Autodesk Inventor part; units mm, degrees
ref_plane "YZ Plane" through (0, 0, 0) normal (1, 0, 0) x (0, 1, 0)
ref_plane "XZ Plane" through (0, 0, 0) normal (0, 1, 0) x (-1, 0, 0)
ref_plane "Arbeitsebene1" through (0, 0, -17.5) normal (0, 0, 1) x (1, 0, 0)
sketch "Skizze1" plane through (0, 0, -17.5) normal (0, 0, 1) x (1, 0, 0)
  arc A0 (5.2, -17) -> (15.2, -17) centre (10.2, -17) ccw
  circle A1 centre (10.2, -17) radius 2.3
  circle A2 centre (10.2, 17) radius 2.3
  arc A3 (15.2, 17) -> (5.2, 17) centre (10.2, 17) ccw
  line L0 (15.2, 17) -> (15.2, -17)
  line L1 (5.2, -17) -> (5.2, 17)
  point P0 (0, 0)
  dimension "d17" = 34
  dimension "d19" = 5
  dimension "d20" = 5
  dimension "d21" = 4.6
  dimension "d22" = 4.6
  dimension "d23" = 5.2
  dimension "d24" = 15.2
  dimension "d25" = 17
extrude "Extrusion1" add sketch "Skizze1" against normal blind 20
sketch "Skizze2" plane through (15.2, -17, -17.5) normal (1, 0, 0) x (0, 0, -1)
  circle A0 centre (-2.1, 17) radius 13.4
  circle A1 centre (-2.1, 17) radius 16.4
  line L0 (0, 39) -> (20, 39)
  line L1 (7, 39) -> (7, 30.6437)
  line L2 (7, 39) -> (-2.3022, 41.2587)
  line L3 (-2.3022, 41.2587) -> (-4.5237, 40.7441)
  line L4 (-4.5237, 40.7441) -> (-5.04, 30.0735)
  line L5 (-5.1067, 3.9417) -> (-12.3463, -18.8233)
  line L6 (-12.3463, -18.8233) -> (7.5061, -24.3836)
  line L7 (7.5061, -24.3836) -> (7, -5)
  line L8 (0, -5) -> (20, -5)
  line L9 (7, -5) -> (7, 3.3563)
  line L10 (0, 0) -> (0, -5)
  line L11 (36.0228, 70.8555) -> (-22.3921, 70.8555)
  line L12 (-22.3921, 70.8555) -> (-22.3921, -28.3632)
  line L13 (-22.3921, -28.3632) -> (36.0228, -28.3632)
  line L14 (36.0228, -28.3632) -> (36.0228, 70.8555)
  point P0 (-17.5, 17)
  point P1 (-6.0183, 1.075)
  point P2 (-4.8906, 33.1608)
  dimension "d5" = 3
  dimension "d6" = 7
  dimension "d26" = 44
  dimension "d27" = 22
  dimension "d28" = 26.8
  dimension "d29" = 15.4
extrude "Extrusion2" cut sketch "Skizze2" against normal blind 10 contours A0 | L14 L13 L12 L11
sketch "Skizze3" plane through (15.2, -17, -24.5) normal (0, 0, -1) x (-1, 0, 0)
  circle A0 centre (5, 34) radius 2.3
  line L0 (2.8638, 30.3) -> (0.7276, 34)
  line L1 (0.7276, 34) -> (2.8638, 37.7)
  line L2 (2.8638, 37.7) -> (7.1362, 37.7)
  line L3 (7.1362, 37.7) -> (9.2724, 34)
  line L4 (9.2724, 34) -> (7.1362, 30.3)
  line L5 (7.1362, 30.3) -> (2.8638, 30.3)
  line L6 (0.7276, 0) -> (2.8638, 3.7)
  line L7 (2.8638, 3.7) -> (7.1362, 3.7)
  line L8 (7.1362, 3.7) -> (9.2724, 0)
  line L9 (9.2724, 0) -> (7.1362, -3.7)
  line L10 (7.1362, -3.7) -> (2.8638, -3.7)
  line L11 (2.8638, -3.7) -> (0.7276, 0)
  point P0 (15.2, 17)
  point P1 (5, 0)
  point P2 (5, 0)
  point P3 (5.6446, 34.7922)
  point P4 (4.3554, 34.7922)
  dimension "d9" = 7.4
  dimension "d10" = 7.4
extrude "Extrusion3" cut sketch "Skizze3" along normal blind 10 and the other way blind 3.5 contours A0 | L0 L1 L2 L3 L4 L5 | L6 L7 L8 L9 L10 L11
fillet "Rundung1" radius 1 2 edges at (15.2, 0, -31.8) (5.2, 0, -31.8)
equation "\"d20\" = d19"
equation "\"d27\" = 0.5 * d26"
equation "\"d10\" = d9"
properties part number "Bracket26_8"
For this review, take the finished solid that the model builds, in its own axes (mm). A direction names the side the tool comes from. Round coordinates to 2 decimals unless told otherwise and drop trailing zeros. Loops run counter-clockwise (first coordinate to the right, second up) from the corner with the lowest first, then second, coordinate; pieces in that order, holes last. Notation, with made-up numbers: (1, -20) - (46, -20) arc R19 cw to (46, 16) - close; hole circle Ø3 at (28.5, 68.5). An arc over 180 degrees is marked (long way). Put each result on its own line as item: value. Start each with the question number.
1. Consider section B-B on x = 10.2. State the section outline as (y, z) points.
2. Insertion check: P1, Ø5.5, axis at x = 10.2, y = -17, coming from the -Z side; P2, Ø1, axis at x = 7.5, z = -24, coming from the -Y side; P3, Ø4, axis at x = 6.5, y = 4, coming from the +Z side. Each pin has a flat end and moves straight along its axis. Give the tip position at first contact, or say it passes through.
3. For probe 1 along Y at (x, z) = (10.2, -20.1); probe 2 along Y at (x, z) = (11.75, -23.25); probe 3 along X at (y, z) = (-19, -22.25), list the stretches that pass through material, from the lowest coordinate up. Write a range as [from, to].
4. Consider section C-C on z = -22. State the section outline as (x, y) points.
5. Consider section A-A on z = -18.5. State the section outline as (x, y) points, plus the area to 3 significant figures.
6. Consider section D-D on x = 7. State the section outline as (y, z) points, plus the area to 3 significant figures.
7. For faces 4 (the cylindrical face through (10.1, -22, -21)), 5 (the flat face through (13.389, 15.124, -23.026)), list the 3-axis set-ups (+Z, -Z, +X, -X, +Y, -Y) from which the entire face can be reached by the end or side of a thin tool; tool diameter is ignored.
8. Mouldability with a two-part tool opening along Y and no side actions: class faces 1 (the flat face through (10, -20, -17.5)), 2 (the cylindrical face through (10.3, -0.2, -31.8)), 3 (the flat face through (7.011, 18.876, -22.774)) as +Y half, -Y half, draft (parallel to the pull), parting line (faces both ways), or undercut.
Result sheet:
1. outline: (-22, -24.5) - (-20.7, -24.5) - (-20.7, -21) - (-19.3, -21) - (-19.3, -17.5) - (-22, -17.5) - close; (-14.7, -21) - (-13.3, -21) - (-13.3, -25) arc R16.4 ccw to (13.3, -25) - (13.3, -21) - (14.7, -21) - (14.7, -17.5) - (13.23, -17.5) arc R13.4 cw to (-13.23, -17.5) - (-14.7, -17.5) - close; (19.3, -21) - (20.7, -21) - (20.7, -24.5) - (22, -24.5) - (22, -17.5) - (19.3, -17.5) - close
2. P1: z = -21
2. P2: y = -21.49
2. P3: z = -27.38
3. probe 1: [-22, -19.3], [-14.7, -12.55], [12.55, 14.7], [19.3, 22]
3. probe 2: [-21.75, -20.7], [-13.3, -10.86], [10.86, 13.3], [20.7, 21.75]
3. probe 3: [5.62, 7.08], [13.32, 14.78]
4. outline: (5.2, -17) arc R5 ccw to (15.2, -17) - (15.2, -11.66) - (5.2, -11.66) - close; (5.2, 11.66) - (15.2, 11.66) - (15.2, 17) arc R5 ccw to (5.2, 17) - close; hole (5.93, -17) - (8.06, -20.7) - (12.34, -20.7) - (14.47, -17) - (12.34, -13.3) - (8.06, -13.3) - close; hole (5.93, 17) - (8.06, 13.3) - (12.34, 13.3) - (14.47, 17) - (12.34, 20.7) - (8.06, 20.7) - close
5. outline: (5.2, -17) arc R5 ccw to (15.2, -17) - (15.2, -13.04) - (5.2, -13.04) - close; (5.2, 13.04) - (15.2, 13.04) - (15.2, 17) arc R5 ccw to (5.2, 17) - close; hole circle Ø4.6 at (10.2, -17); hole circle Ø4.6 at (10.2, 17)
5. area: 125 mm^2
6. outline: (-20.84, -24.5) - (-18.86, -24.5) - (-18.86, -21) - (-15.14, -21) - (-15.14, -24.5) - (-13.64, -24.5) arc R16.4 ccw to (13.64, -24.5) - (15.14, -24.5) - (15.14, -21) - (18.86, -21) - (18.86, -24.5) - (20.84, -24.5) - (20.84, -17.5) - (13.23, -17.5) arc R13.4 cw to (-13.23, -17.5) - (-20.84, -17.5) - close
6. area: 180 mm^2
7. face 4: +Z, -Z, -Y
7. face 5: -Z
8. face 1: draft
8. face 2: parting line
8. face 3: undercut
